```python
from build123d import *

# Parameters (mm, degrees)
EXTRUDE004_DEPTH = 30
PAD008_DEPTH     = 50


with BuildPart() as bearingslot001:
    # Sketch025 → Extrude004 (new body)
    with BuildSketch(Plane.XY):
        with BuildLine():
            ThreePointArc((-5.33868, 5.338632), (0, -7.55), (5.33868, 5.338632))
            Line((1.5, 9.177312), (5.33868, 5.338632))
            Line((1.5, 17), (1.5, 9.177312))
            Line((-1.5, 17), (1.5, 17))
            Line((-1.5, 9.177312), (-1.5, 17))
            Line((-5.33868, 5.338632), (-1.5, 9.177312))
        make_face()
    extrude(amount=EXTRUDE004_DEPTH)


with BuildPart() as bearingslot001_1:
    # Extrude004 placement: moved
    add(bearingslot001.part.moved(Location((0, 0, 3))))


with BuildPart() as obj1:
    # Sketch024 → Pad008 (new body)
    with BuildSketch(Plane.XY):
        with BuildLine():
            ThreePointArc((-3.535534, 3.535534), (0, -5), (3.535534, 3.535534))
            Line((1.5, 5.571068), (3.535534, 3.535534))
            Line((1.5, 17), (1.5, 5.571068))
            Line((-1.5, 17), (1.5, 17))
            Line((-1.5, 5.571068), (-1.5, 17))
            Line((-3.535534, 3.535534), (-1.5, 5.571068))
        make_face()
    extrude(amount=PAD008_DEPTH)

    # Fusion002: union BearingSlot001
    add(bearingslot001_1.part)


solid = obj1.part
```
Verification items for the finished model (mm, model axes). A direction names the side the tool comes from. Coordinates: 2 decimals unless noted, no trailing zeros. Write each loop counter-clockwise with the first axis right and the second up, starting at its lowest first coordinate (ties: lowest second). Pieces come first, ordered by that corner, then holes. Notation, with made-up numbers: M 59.5,64.5 L 109.5,64.5 A24 ccw 109.5,97.5 Z; hole C 21.25,42.5 d4. An arc over 180 degrees is marked long. One line per item, written item: value.
Item 1: Scan lines: line 1 along X through (y, z) = (10.75, 7.5); line 2 along Z through (x, y) = (1.75, 7.5); line 3 along Y through (x, z) = (2.75, 27.5). Record each from-to range of solid material in increasing order.
Check sheet entries:
line 1: x = -1.5 to 1.5
line 2: z = 3 to 33
line 3: y = -7.03 to 7.93
Item 2: Gauge pin test, flat ends, axial feed: pin 1 Ø9 at (y, z) = (13, 20.5) entering from -X; pin 2 Ø2 at (y, z) = (-2, 30) entering from +X; pin 3 Ø3.5 at (y, z) = (9.5, 29) entering from +X. Record the tip position at first contact, or that the pin passes through.
Check sheet entries:
pin 1: stops at x = -2.18
pin 2: stops at x = 7.48
pin 3: stops at x = 2.93
Item 3: Section check C-C, the plane y = 0. Record the boundary of the cut face in (x, z).
Check sheet entries:
outline: M -7.55,3 L -5,3 L -5,0 L 5,0 L 5,3 L 7.55,3 L 7.55,33 L 5,33 L 5,50 L -5,50 L -5,33 L -7.55,33 Z
Item 4: Section check B-B, the plane x = 0. Record the boundary of the cut face in (y, z).
Check sheet entries:
outline: M -7.55,3 L -5,3 L -5,0 L 17,0 L 17,50 L -5,50 L -5,33 L -7.55,33 Z
Item 5: Access from +Z, -Z, +X, -X, +Y, -Y to the whole of each face (thin tool, end or side, straight path). Record for faces 1 (the flat face through (2.5, 4.57, 1.48)), 2 (the flat face through (2.5, 4.57, 41.38)), 3 (the cylindrical face through (0, -5, 41)), 4 (the cylindrical face through (0, -5, 1)), 5 (the flat face through (-2.53, 4.54, 41.38)).
Check sheet entries:
face 1: -Z, +X, +Y
face 2: +Z, +X, +Y
face 3: +Z
face 4: -Z
face 5: +Z, -X, +Y
Item 6: Section check A-A, the plane z = 6. Record the boundary of the cut face in (x, y).
Check sheet entries:
outline: M -5.34,5.34 A7.55 ccw long 5.34,5.34 L 1.5,9.18 L 1.5,17 L -1.5,17 L -1.5,9.18 Z
Item 7: Section check D-D, the plane y = 8.5. Record the boundary of the cut face in (x, z).
Check sheet entries:
outline: M -2.18,3 L -1.5,3 L -1.5,0 L 1.5,0 L 1.5,3 L 2.18,3 L 2.18,33 L 1.5,33 L 1.5,50 L -1.5,50 L -1.5,33 L -2.18,33 Z
